Check sheet for the modelled part. Datum: model origin and axes. Units: mm. A direction names the side the tool comes from. Round coordinates to 2 decimals unless told otherwise and drop trailing zeros. Order: outer loops, then holes, each group sorted by start corner. A loop starts at its lowest first (then second) coordinate and runs counter-clockwise, first axis right, second up. Notation, with made-up numbers: (88.25, -21.75) -> (131.25, -21.75) arc R16 cw to (131.25, -12.75) -> close; hole circle Ø1 at (80, 28). An arc over 180 degrees is marked (long way). Answer in a Markdown table with one row per item. Add a question column.
1. Sectioned sample at A-A, the plane y = -42. Record the boundary of the cut face in (x, z), then the cut area to 3 significant figures.
2. Sectioned sample at C-C, the plane y = 55. Record the boundary of the cut face in (x, z), then the cut area to 3 significant figures.
3. Access from +Z, -Z, +X, -X, +Y, -Y to the whole of each face (thin tool, end or side, straight path). Record for faces 3 (the flat face through (-124, -76.5, 0)), 4 (the flat face through (-125, 23, -5)).
4. Draft check along Y on faces 1 (the flat face through (-122, -83, -1)), 2 (the flat face through (-125, 9, -22)). Enter one of: +Y half, -Y half, draft (parallel to the pull), parting line (faces both ways), or undercut.
5. Sectioned sample at B-B, the plane x = -120. Count the separate pieces of the cut face and the enclosed holes in it, then the cut area to 3 significant figures.
6. Material ranges on L1, parallel to Z at x = -127, y = 41; L2, parallel to Y at x = -120, z = -38.05; L3, parallel to Z at x = -126.75, y = 23, recorded low to high. Write a range as from..to.
7. Depth check by flat-ended pin: P1, Ø1, axis at y = -53.5, z = 1.5, coming from the +X side. Enter the tip coordinate at first touch or a pass-through.
```python
from build123d import *

# Parameters (mm, degrees)
SKETCH008_W     = 166
SKETCH008_H     = 80
PAD005_DEPTH    = 12
SKETCH009_W     = 160.5
SKETCH009_H     = 73.5
POCKET002_DEPTH = 9
SKETCH016_W     = 153
SKETCH016_H     = 63
PAD007_DEPTH    = 4
SKETCH012_R     = 1.4
SKETCH012_W     = 70
SKETCH012_H     = 12.5
SKETCH012_W_2   = 50
SKETCH012_H_2   = 28
SKETCH012_W_3   = 12
SKETCH012_H_3   = 3
POCKET008_DEPTH = 12.001
SKETCH023_R     = 1.75
POCKET011_DEPTH = 80.001
SKETCH039_W     = 32
SKETCH039_H     = 52
POCKET036_DEPTH = 2
CHAMFER033_SIZE = 1
POCKET038_DEPTH = 154


with BuildPart() as part:
    # Sketch008 → Pad005 (new body)
    with BuildSketch(Plane.YZ):
        Rectangle(SKETCH008_W, SKETCH008_H)
    extrude(amount=PAD005_DEPTH)

    # Sketch009 (on Face6 of Pad005) → Pocket002 (cut)
    with BuildSketch(Plane.YZ.offset(12)):
        Rectangle(SKETCH009_W, SKETCH009_H)
    extrude(amount=-POCKET002_DEPTH, mode=Mode.SUBTRACT)

    # Sketch016 (on Face11 of Pocket002) → Pad007 (join)
    with BuildSketch(Plane.YZ.offset(3)):
        Rectangle(SKETCH016_W, SKETCH016_H)
    extrude(amount=PAD007_DEPTH)

    # Sketch012 (on Face4 of Pocket002) → Pocket008 (cut, through all)
    with BuildSketch(Plane(origin=(0, 0, 0), x_dir=(0, 1, 0), z_dir=(-1, 0, 0))):
        with Locations((23, 11)):
            Circle(SKETCH012_R)
        with Locations((23, -29)):
            Circle(SKETCH012_R)
        with Locations((-70, 28)):
            Circle(SKETCH012_R)
        with Locations((-70, 9)):
            Circle(SKETCH012_R)
        with Locations((-10, 28)):
            Circle(SKETCH012_R)
        with Locations((-10, 9)):
            Circle(SKETCH012_R)
        with Locations((-40, 18.5)):
            Rectangle(SKETCH012_W, SKETCH012_H)
        with Locations((23, -9)):
            Rectangle(SKETCH012_W_2, SKETCH012_H_2)
        with Locations((9, 26.5)):
            Rectangle(SKETCH012_W_3, SKETCH012_H_3)
        with Locations((26, 26.5)):
            Rectangle(SKETCH012_W_3, SKETCH012_H_3)
        with Locations((43, 26.5)):
            Rectangle(SKETCH012_W_3, SKETCH012_H_3)
        with Locations((9, 20.5)):
            Rectangle(SKETCH012_W_3, SKETCH012_H_3)
        with Locations((26, 20.5)):
            Rectangle(SKETCH012_W_3, SKETCH012_H_3)
        with Locations((43, 20.5)):
            Rectangle(SKETCH012_W_3, SKETCH012_H_3)
        with Locations((63.63, 21)):
            Rectangle(SKETCH012_W_3, SKETCH012_H_3)
        with Locations((63.63, 15)):
            Rectangle(SKETCH012_W_3, SKETCH012_H_3)
        with Locations((63.63, 9)):
            Rectangle(SKETCH012_W_3, SKETCH012_H_3)
        with Locations((63.63, 3)):
            Rectangle(SKETCH012_W_3, SKETCH012_H_3)
        with Locations((63.63, -3)):
            Rectangle(SKETCH012_W_3, SKETCH012_H_3)
        with Locations((63.63, -9)):
            Rectangle(SKETCH012_W_3, SKETCH012_H_3)
        with Locations((63.63, -15)):
            Rectangle(SKETCH012_W_3, SKETCH012_H_3)
        with Locations((63.63, -21)):
            Rectangle(SKETCH012_W_3, SKETCH012_H_3)
    extrude(amount=-POCKET008_DEPTH, mode=Mode.SUBTRACT)

    # Sketch023 (on Face1 of Pocket008) → Pocket011 (cut, through all)
    with BuildSketch(Plane(origin=(0, 0, 40), x_dir=(0, -1, 0), z_dir=(0, 0, 1))):
        with Locations((-65, 8.5)):
            Circle(SKETCH023_R)
        with Locations((65, 8.5)):
            Circle(SKETCH023_R)
        with Locations((0, 8.5)):
            Circle(SKETCH023_R)
    extrude(amount=-POCKET011_DEPTH, mode=Mode.SUBTRACT)

    # Sketch039 → Pocket036 (cut)
    with BuildSketch(Plane.YZ.offset(7)):
        with Locations((60, 0)):
            Rectangle(SKETCH039_W, SKETCH039_H)
    extrude(amount=-POCKET036_DEPTH, mode=Mode.SUBTRACT)

    # Chamfer033
    chamfer033_edges = [part.edges().sort_by_distance(p)[0] for p in [
        (6, -83, 40),
        (6, 83, 40),
        (6, -83, -40),
        (6, 83, -40),
        (0, 83, 0),
        (0, 0, -40),
        (0, -83, 0),
        (0, 0, 40),
    ]]
    chamfer(chamfer033_edges, length=CHAMFER033_SIZE)

    # Sketch056 (on Face103 of Chamfer033) → Pocket038 (cut)
    with BuildSketch(Plane(origin=(0, -76.5, 0), x_dir=(0, 0, -1), z_dir=(0, -1, 0))):
        Polygon((-31.764254, 4.395752), (-28.984535, 7.542603), (-32.262505, 7.752388), align=None)
    extrude(amount=-POCKET038_DEPTH, mode=Mode.SUBTRACT)


with BuildPart() as part_1:
    # Body004 placement: moved
    add(part.part.moved(Location((-128.5, 0, 0))))


solid = part_1.part
```
Answer key:
| question | item | result |
|---|---|---|
| 1 | outline | (-128.5, -39) -> (-127.5, -40) -> (-116.5, -40) -> (-116.5, -36.75) -> (-125.5, -36.75) -> (-125.5, -31.5) -> (-121.5, -31.5) -> (-121.5, -24.75) -> (-128.5, -24.75) -> close; (-128.5, -12.25) -> (-121.5, -12.25) -> (-121.5, 29.46) -> (-123.81, 31.5) -> (-125.5, 31.5) -> (-125.5, 36.75) -> (-116.5, 36.75) -> (-116.5, 40) -> (-127.5, 40) -> (-128.5, 39) -> close |
| 1 | area | 460 mm² |
| 2 | outline | (-128.5, -39) -> (-127.5, -40) -> (-116.5, -40) -> (-116.5, -36.75) -> (-125.5, -36.75) -> (-125.5, -31.5) -> (-121.5, -31.5) -> (-121.5, -26) -> (-123.5, -26) -> (-123.5, 26) -> (-121.5, 26) -> (-121.5, 29.46) -> (-123.81, 31.5) -> (-125.5, 31.5) -> (-125.5, 36.75) -> (-116.5, 36.75) -> (-116.5, 40) -> (-127.5, 40) -> (-128.5, 39) -> close |
| 2 | area | 443 mm² |
| 3 | face 3 | +X |
| 3 | face 4 | +X, -X |
| 4 | face 1 | -Y half |
| 4 | face 2 | undercut |
| 5 | separate pieces | 6 |
| 5 | enclosed holes | 0 |
| 5 | area | 1,410 mm² |
| 6 | L1 | z = -40..-28, -25..-22, -19..-5, 23..40 |
| 6 | L2 | y = -83..-66.75, -63.25..-1.75, 1.75..63.25, 66.75..83 |
| 6 | L3 | z = -40..-28, -25..-22, -19..-12.4, -9.6..-5, 23..27.6, 30.4..40 |
| 7 | P1 | stops at x = -121.5 |
